Read the model definition and answer for the solid it produces. Units are mm, in the model's axes. A direction names the side the tool comes from. Round coordinates to 2 decimals unless told otherwise and drop trailing zeros. Write each loop counter-clockwise with the first axis right and the second up, starting at its lowest first coordinate (ties: lowest second). Pieces come first, ordered by that corner, then holes. Notation, with made-up numbers: (15.25, 35) -> (55.25, 35) arc R29 ccw to (55.25, 61) -> close; hole circle Ø8 at (-40, 8.5). An arc over 180 degrees is marked (long way). Return JSON: item names as keys, results as strings. Group by question number.
(1) A cutting plane is placed at C-C on x = 0. Give the vertices of the cut face in (y, z).
(2) A cutting plane is placed at A-A on y = -11.5. Give the vertices of the cut face in (x, z).
(3) The mould has two halves that part along X. Classify faces 1 (the flat face through (0, -11, -17.5)), 2 (the flat face through (-11.5, -4, -2)), 3 (the cylindrical face through (10.9, 13.43, -0.04)), 4 (the cylindrical face through (9.02, 3.96, -0.04)): released by +X, released by -X, zero draft, split by the parting line, or undercut.
(4) Straight lines are drawn through the part: line 1 (Y direction, x = 0, z = 1.5); line 2 (Z direction, x = 0, y = -11); line 3 (X direction, y = -1, z = 0.4). For each, find the intervals that lie inside material, in ascending order.
(5) For faces 5 (the cylindrical face through (-0.145, 11.247, -0.035)), 6 (the flat face through (0, 3, -2.5)), 7 (the flat face through (0, -14, -7)), determine the directions among +Z, -Z, +X, -X, +Y, -Y from which every point of the face is accessible in a straight line to the end or side of a thin tool.
(6) A cutting plane is placed at B-B on z = -1.5. Give the vertices of the cut face in (x, y), then the cut area to 3 significant figures.
(7) A cutting plane is placed at D-D on y = -1. Give the vertices of the cut face in (x, z), then the cut area to 3 significant figures.
(8) Given pin 1 (7 mm diameter, centred on x = 0, z = -10, fed in from +Y); pin 2 (1 mm diameter, centred on x = -6.5, y = 8.5, fed in from -Z); pin 3 (6 mm diameter, centred on x = 5, y = 9, fed in from -Z), each flat-ended and moving along its own axis, determine where each tip first touches the part or whether it passes through.
Autodesk Inventor part; units mm, degrees
ref_plane "YZ Plane" through (0, 0, 0) normal (1, 0, 0) x (0, 1, 0)
ref_plane "XZ Plane" through (0, 0, 0) normal (0, 1, 0) x (-1, 0, 0)
ref_plane "XY Plane" through (0, 0, 0) normal (0, 0, 1) x (1, 0, 0)
sketch "Sketch1" plane through (0, 0, 0) normal (0, 0, 1) x (1, 0, 0)
  line L0 (-11.5, -14) -> (11.5, -14)
  line L1 (11.5, -14) -> (11.5, 14)
  line L2 (11.5, 14) -> (-11.5, 14)
  line L3 (-11.5, 14) -> (-11.5, -14)
  line L4 (-11.5, -14) -> (11.5, 14) construction
  line L5 (11.5, -14) -> (-11.5, 14) construction
  point P0 (0, 0)
  dimension "d0" = 23
  dimension "d1" = 28
extrude "Extrusion1" add sketch "Sketch1" along normal mid plane 5
sketch "Sketch2" plane through (0, 0, -2.5) normal (0, 0, -1) x (-1, 0, 0)
  line L0 (11.5, -14) -> (-11.5, -14)
  line L1 (-11.5, -14) -> (11.5, -14)
  line L2 (11.5, -14) -> (11.5, -9)
  line L3 (11.5, -9) -> (-11.5, -9)
  line L4 (-11.5, -9) -> (-11.5, -14)
  line L5 (11.5, -14) -> (11.5, 14)
  point P0 (0, 0)
  dimension "d4" = 5
extrude "Extrusion2" add sketch "Sketch2" along normal blind 15
sketch "Sketch3" plane through (-11.5, -9, -2.5) normal (0, 1, 0) x (1, 0, 0)
  line L0 (0, 0) -> (0, 15)
  line L1 (0, 15) -> (23, 15)
  point P0 (11.5, -2.5)
  point P1 (11.5, 7.5)
  point P2 (0, 7.5)
  point P3 (11.5, 15)
hole "Hole1" at (0, -9, -10) direction (0, -1, 0) diameter 4.496 end through all
sketch "Sketch4" plane through (0, 0, -2.5) normal (0, 0, -1) x (-1, 0, 0)
  line L0 (11.5, 14) -> (-11.5, 14)
  line L1 (11.5, -9) -> (-11.5, -9)
  point P0 (0, 0)
  point P1 (0, -1)
  point P2 (0, 14)
  dimension "d14" = 8
hole "Hole2" at (0, -1, -2.5) direction (0, 0, 1) diameter 4.496 end through all
sketch "Sketch5" plane through (0, 0, -2.5) normal (0, 0, -1) x (-1, 0, 0)
  circle A0 centre (0, -1) radius 10 construction
  arc A1 (-9.186, 7.1013) -> (-5.814, 4.1275) centre (-7.5, 5.6144) ccw
  arc A2 (5.814, 4.1275) -> (9.186, 7.1013) centre (7.5, 5.6144) ccw
  arc A3 (9.186, 7.1013) -> (-9.186, 7.1013) centre (0, -1) ccw
  arc A4 (5.814, 4.1275) -> (-5.814, 4.1275) centre (0, -1) ccw
  line L0 (-7.5, 5.6144) -> (7.5, 5.6144) construction
  line L1 (-11.5, 14) -> (-11.5, -9) construction
  circle A5 centre (0, -1) radius 2.248
  point P0 (0, 5.6144)
  dimension "d22" = 20
  dimension "d23" = 4.496
  dimension "d24" = 4
extrude "Extrusion3" cut sketch "Sketch5" against normal through all contours A3 A2 A4 A1
fillet "Fillet1" radius 2 4 edges at (11.5, 14, 0) (-11.5, 14, 0) (11.5, -11.5, -17.5) (-11.5, -11.5, -17.5)
properties part number "RotateLBracket"
Checks:
{
 "1": {"outline": "(-14, -17.5) -> (-9, -17.5) -> (-9, -12.25) -> (-14, -12.25) -> close; (-14, -7.75) -> (-9, -7.75) -> (-9, -2.5) -> (-3.25, -2.5) -> (-3.25, 2.5) -> (-14, 2.5) -> close; (1.25, -2.5) -> (6.75, -2.5) -> (6.75, 2.5) -> (1.25, 2.5) -> close; (11.25, -2.5) -> (14, -2.5) -> (14, 2.5) -> (11.25, 2.5) -> close"},
 "2": {"outline": "(-11.5, -15.5) arc R2 ccw to (-9.5, -17.5) -> (9.5, -17.5) arc R2 ccw to (11.5, -15.5) -> (11.5, 2.5) -> (-11.5, 2.5) -> close; hole circle Ø4.5 at (0, -10)"},
 "3": {"face 1": "zero draft", "face 2": "released by -X", "face 3": "released by +X", "face 4": "undercut"},
 "4": {"line 1": "y = -14 to -3.25, 1.25 to 6.75, 11.25 to 14", "line 2": "z = -17.5 to -12.25, -7.75 to 2.5", "line 3": "x = -11.5 to -2.25, 2.25 to 11.5"},
 "5": {"face 5": "+Z, -Z", "face 6": "-Z, +X, -X, +Y", "face 7": "+Z, -Z, +X, -X, -Y"},
 "6": {"outline": "(-11.5, -14) -> (11.5, -14) -> (11.5, 12) arc R2 ccw to (9.5, 14) -> (-9.5, 14) arc R2 ccw to (-11.5, 12) -> close; hole (-9.19, 7.1) arc R2.25 ccw to (-5.81, 4.13) arc R7.75 cw to (5.81, 4.13) arc R2.25 ccw to (9.19, 7.1) arc R12.25 ccw to start; hole circle Ø4.5 at (0, -1)", "area": "534 mm^2"},
 "7": {"outline": "(-11.5, -2.5) -> (-2.25, -2.5) -> (-2.25, 2.5) -> (-11.5, 2.5) -> close; (2.25, -2.5) -> (11.5, -2.5) -> (11.5, 2.5) -> (2.25, 2.5) -> close", "area": "92.5 mm^2"},
 "8": {"pin 1": "stops at y = -9", "pin 2": "passes through", "pin 3": "stops at z = -2.5"}
}
